```python
from build123d import *

# Parameters (mm, degrees)
ESQUISSE1_W             = 44.6
ESQUISSE1_H             = 36
ESQUISSE1_W_2           = 25.4
BOSS_EXTRU_1_DEPTH      = 5
ESQUISSE2_W             = 25.4
ESQUISSE2_H             = 3
BOSS_EXTRU_2_DEPTH      = 5.6
ESQUISSE3_W             = 40
ESQUISSE3_H             = 36
BOSS_EXTRU_4_DEPTH      = 15
ENL_V_MAT_EXTRU_3_DEPTH = 60.246603278
ESQUISSE7_W             = 20
ESQUISSE7_H             = 8
ENL_V_MAT_EXTRU_4_DEPTH = 61.70551886
CONG_4_R                = 0.5


with BuildPart() as part:
    # Esquisse1 → Boss.-Extru.1 (new body)
    with BuildSketch(Plane.XY):
        with Locations((-22.3, 18)):
            Rectangle(ESQUISSE1_W, ESQUISSE1_H)
        with Locations((12.7, 18)):
            Rectangle(ESQUISSE1_W_2, ESQUISSE1_H)
    extrude(amount=BOSS_EXTRU_1_DEPTH)

    # Esquisse2 → Boss.-Extru.2 (add)
    with BuildSketch(Plane(origin=(0, 0, 0), x_dir=(-1, 0, 0), z_dir=(0, 0, -1))):
        with Locations((-12.7, 1.5)):
            Rectangle(ESQUISSE2_W, ESQUISSE2_H)
        with Locations((-12.7, 34.5)):
            Rectangle(ESQUISSE2_W, ESQUISSE2_H)
    extrude(amount=BOSS_EXTRU_2_DEPTH)

    # Esquisse3 → Boss.-Extru.4 (add)
    with BuildSketch(Plane(origin=(0, 0, 0), x_dir=(-1, 0, 0), z_dir=(0, 0, -1))):
        with Locations((24.6, 18)):
            Rectangle(ESQUISSE3_W, ESQUISSE3_H)
    extrude(amount=BOSS_EXTRU_4_DEPTH)

    # Esquisse4 → Enlèv. mat.-Extru.3 (cut, through all)
    with BuildSketch(Plane(origin=(0, 36, 0), x_dir=(1, 0, 0), z_dir=(0, 1, 0))):
        with BuildLine():
            Line((-24.6, 10), (-44.6, 10))
            Line((-44.6, 10), (-44.6, -5))
            Line((-44.6, -5), (-9.6, -5))
            Line((-9.6, -5), (-5.318745152, -5))
            add(Edge.make_bspline(
                [(-24.6, 10), (-18.581113582, 10.250438225), (-16.538607269, -4.688596284), (-5.318745152, -5)],
                knots=[0, 0, 0, 0, 0.979442109, 0.979442109, 0.979442109, 0.979442109], degree=3))
        make_face()
        with BuildLine():
            Line((-4.6, 15), (-24.6, 15))
            add(Edge.make_bspline(
                [(-4.6, 0), (-13.772339743, 0.318713019), (-15.546263661, 14.974819889), (-24.6, 15)],
                knots=[0, 0, 0, 0, 1, 1, 1, 1], degree=3))
            Line((-4.6, 0), (-4.6, 15))
        make_face()
    extrude(amount=-ENL_V_MAT_EXTRU_3_DEPTH, mode=Mode.SUBTRACT)

    # Esquisse7 → Enlèv. mat.-Extru.4 (cut, through all)
    with BuildSketch(Plane(origin=(0, 0, -15), x_dir=(-1, 0, 0), z_dir=(0, 0, -1))):
        with Locations((34.6, 4)):
            Rectangle(ESQUISSE7_W, ESQUISSE7_H)
        with BuildLine():
            Line((24.6, 0), (24.6, 8))
            add(Edge.make_bspline(
                [(0.1, 0), (6.766666667, 0), (17.933333333, 8), (24.6, 8)],
                knots=[0, 0, 0, 0, 1, 1, 1, 1], degree=3))
            Line((0.1, 0), (24.6, 0))
        make_face()
        with BuildLine():
            add(Edge.make_bspline(
                [(24.6, 28), (17.933333333, 28), (6.766666667, 36), (0.1, 36)],
                knots=[0, 0, 0, 0, 1, 1, 1, 1], degree=3))
            Line((24.6, 28), (24.6, 36))
            Line((24.6, 36), (0.1, 36))
        make_face()
        with Locations((34.6, 32)):
            Rectangle(ESQUISSE7_W, ESQUISSE7_H)
    extrude(amount=-ENL_V_MAT_EXTRU_4_DEPTH, mode=Mode.SUBTRACT)

    # Congé4
    cong_4_edges = [part.edges().sort_by_distance(p)[0] for p in [
        (-15.717570787, 30.513571579, -1.106703523),
        (-44.6, 28, -12.5),
        (-2.74987965, 35.666138518, 5),
        (12.65, 0, 5),
        (25.4, 18, 5),
        (12.65, 36, 5),
        (-44.6, 18, -10),
        (-34.6, 28, -10),
        (-34.6, 8, -10),
        (-15.717570798, 5.486428428, -1.10670351),
        (-44.6, 8, -12.5),
        (-2.749879652, 0.333861473, 5),
    ]]
    fillet(cong_4_edges, radius=CONG_4_R)


solid = part.part
```
Can you work these out from the model? Positions are in its coordinate system, mm. A direction names the side the tool comes from. Coordinates: 2 decimals unless noted, no trailing zeros. Write each loop counter-clockwise with the first axis right and the second up, starting at its lowest first coordinate (ties: lowest second). Pieces come first, ordered by that corner, then holes. Notation, with made-up numbers: (24.25, 32.25) - (41.25, 32.25) arc R17 cw to (41.25, 37.25) - close; hole circle Ø10 at (38.5, -32.75). An arc over 180 degrees is marked (long way). Return JSON: item names as keys, results as strings.
Q1. On a 3-axis mill with a long thin cutter (end or side, diameter ignored), from which of +Z, -Z, +X, -X, +Y, -Y can I reach the whole of each face in a straight line? I mean faces 1 (the flat face through (13, 33, -3)), 2 (the flat face through (-34, 8, -13)), 3 (the flat face through (13, 35, -5.6)), 4 (the flat face through (-34, 18, -10)), 5 (the flat face through (-34, 28, -13)). Say none if no direction works.
Computed values:
{"face 1": "-Z, +X", "face 2": "+Z, -Z, -X, -Y", "face 3": "-Z, +X, -X, +Y, -Y", "face 4": "+Z, -X, +Y, -Y", "face 5": "+Z, -Z, -X, +Y"}
Q2. If we section it at B-B (z = -3.5): Count the separate pieces of the cut face and the enclosed holes in it, then the cut area to 3 significant figures.
Computed values:
{"separate pieces": "3", "enclosed holes": "0", "area": "312 mm2"}
Q3. If we section it at C-C (x = -29.5): Please give me the cut outline in (y, z), then the cut area to 3 significant figures.
Computed values:
{"outline": "(8, -15) - (28, -15) - (28, -10.5) arc R0.5 ccw to (27.5, -10) - (8.5, -10) arc R0.5 ccw to (8, -10.5) - close", "area": "99.9 mm2"}
Q4. If we section it at A-A (x = 11): Please give me the cut outline in (y, z).
Computed values:
{"outline": "(0, -5.6) - (3, -5.6) - (3, 0) - (33, 0) - (33, -5.6) - (36, -5.6) - (36, 4.5) arc R0.5 ccw to (35.5, 5) - (0.5, 5) arc R0.5 ccw to (0, 4.5) - close"}
Q5. Please list where these lines run through material, in increasing order: L1, parallel to Y at x = 21.5, z = -1.25; L2, parallel to Z at x = -1, y = 20.5; L3, parallel to Z at x = -30.5, y = 27.5. Write a range as from..to.
Computed values:
{"L1": "y = 0..3, 33..36", "L2": "z = 0..5", "L3": "z = -15..-10"}
Q6. I'm going to push flat-ended pins straight in: pin 1 Ø1.3 at (x, z) = (-35, -12) entering from -Y; pin 2 Ø12 at (x, z) = (-22.5, -7.5) entering from -Y; pin 3 Ø1.5 at (y, z) = (1.5, -2) entering from -X; pin 4 Ø1.5 at (x, z) = (-36, -7.5) entering from +Y. Where does each tip first touch, or does it pass through?
Computed values:
{"pin 1": "stops at y = 8", "pin 2": "stops at y = 5.82", "pin 3": "stops at x = 0", "pin 4": "passes through"}
